```python
from build123d import *

# Parameters (mm, degrees)
F3_DEPTH = 25.4


with BuildPart() as f1:
    # F0 (on Front) → F1 (revolve)
    with BuildSketch(Plane.XZ):
        with BuildLine():
            Line((0, 25.4), (0, 0))
            Line((0, 0), (25.4, 0))
            Line((25.4, 0), (9.75633, 24.067192))
            ThreePointArc((9.75633, 24.067192), (8.359358, 25.168282), (6.692807, 25.790008))
            Line((6.692807, 25.790008), (7.097861, 76.18158))
            Line((7.097861, 76.18158), (0, 76.18158))
            Line((0, 76.18158), (0, 25.4))
        make_face()
    revolve(axis=Axis((0, 0, 12.7), (0, 0, 1)))

    # F2 (on Top) → F3 (cut)
    with BuildSketch(Plane.XY):
        with BuildLine():
            Line((3.175, -3.175), (3.175, -37.026545))
            ThreePointArc((3.175, -37.026545), (26.277801, -26.277801), (37.026545, -3.175))
            Line((37.026545, -3.175), (3.175, -3.175))
        make_face()
        with BuildLine():
            Line((3.175, 3.175), (37.173723, 3.175))
            ThreePointArc((37.173723, 3.175), (26.381493, 26.381493), (3.175, 37.173723))
            Line((3.175, 37.173723), (3.175, 3.175))
        make_face()
        with BuildLine():
            Line((-3.175, 3.175), (-3.175, 36.787234))
            ThreePointArc((-3.175, 36.787234), (-26.109205, 26.109205), (-36.787234, 3.175))
            Line((-36.787234, 3.175), (-3.175, 3.175))
        make_face()
        with BuildLine():
            Line((-3.175, -3.175), (-37.173723, -3.175))
            ThreePointArc((-37.173723, -3.175), (-26.381493, -26.381493), (-3.175, -37.173723))
            Line((-3.175, -37.173723), (-3.175, -3.175))
        make_face()
    extrude(amount=F3_DEPTH, mode=Mode.SUBTRACT)


solid = f1.part
```
Verification items for the finished model (mm, model axes). A direction names the side the tool comes from. Coordinates: 2 decimals unless noted, no trailing zeros. Write each loop counter-clockwise with the first axis right and the second up, starting at its lowest first coordinate (ties: lowest second). Pieces come first, ordered by that corner, then holes. Notation, with made-up numbers: M -1.75,50 L 31.25,50 A22 ccw 31.25,76 Z; hole C -7.75,58.5 d3. An arc over 180 degrees is marked long. One line per item, written item: value.
Item 1: Scan lines: line 1 along Y through (x, z) = (15, 9) (3 decimals); line 2 along X through (y, z) = (-1.5, 62). Record each from-to range of solid material in increasing order.
Check sheet entries:
line 1: y = -3.175 to 3.175
line 2: x = -6.82 to 6.82
Item 2: Mould release check, pull along Z, two halves, no side actions. Record for faces 4 (the conical face through (6.58, 2.07, 51.34)), 5 (the conical face through (-0.07, -15.73, 14.88)), 6 (the flat face through (12, 3.175, 10)), 7 (the flat face through (-5, -5, 25.4)): pulls with the +Z half, pulls with the -Z half, needs draft (parallel to the pull), parting line crosses it, or undercut.
Check sheet entries:
face 4: undercut
face 5: pulls with the +Z half
face 6: needs draft
face 7: pulls with the -Z half
Item 3: Access from +Z, -Z, +X, -X, +Y, -Y to the whole of each face (thin tool, end or side, straight path). Record for faces 1 (the flat face through (-12, 3.175, 10)), 2 (the flat face through (3.175, -12, 10)), 3 (the flat face through (-3.175, -12, 10)).
Check sheet entries:
face 1: -Z, -X, +Y
face 2: -Z, +X, -Y
face 3: -Z, -X, -Y
Item 4: Section check A-A, the plane z = 13. Record the boundary of the cut face in (x, y) (3 decimals).
Check sheet entries:
outline: M -16.65,-3.175 L -3.175,-3.175 L -3.175,-16.65 A16.95 ccw 3.175,-16.65 L 3.175,-3.175 L 16.65,-3.175 A16.95 ccw 16.65,3.175 L 3.175,3.175 L 3.175,16.65 A16.95 ccw -3.175,16.65 L -3.175,3.175 L -16.65,3.175 A16.95 ccw Z
Item 5: Section check B-B, the plane z = 51. Record the boundary of the cut face in (x, y).
Check sheet entries:
outline: C 0,0 d13.79
Item 6: Gauge pin test, flat ends, axial feed: pin 1 Ø5 at (y, z) = (-11, 20) entering from -X (3 decimals); pin 2 Ø17.5 at (y, z) = (-16.5, 10.5) entering from +X (3 decimals); pin 3 Ø1 at (x, z) = (4, 65.5) entering from -Y; pin 4 Ø5 at (x, y) = (9.5, -7) entering from -Z. Record the tip position at first contact, or that the pin passes through.
Check sheet entries:
pin 1: stops at x = -3.175
pin 2: stops at x = 3.175
pin 3: stops at y = -6.08
pin 4: passes through
